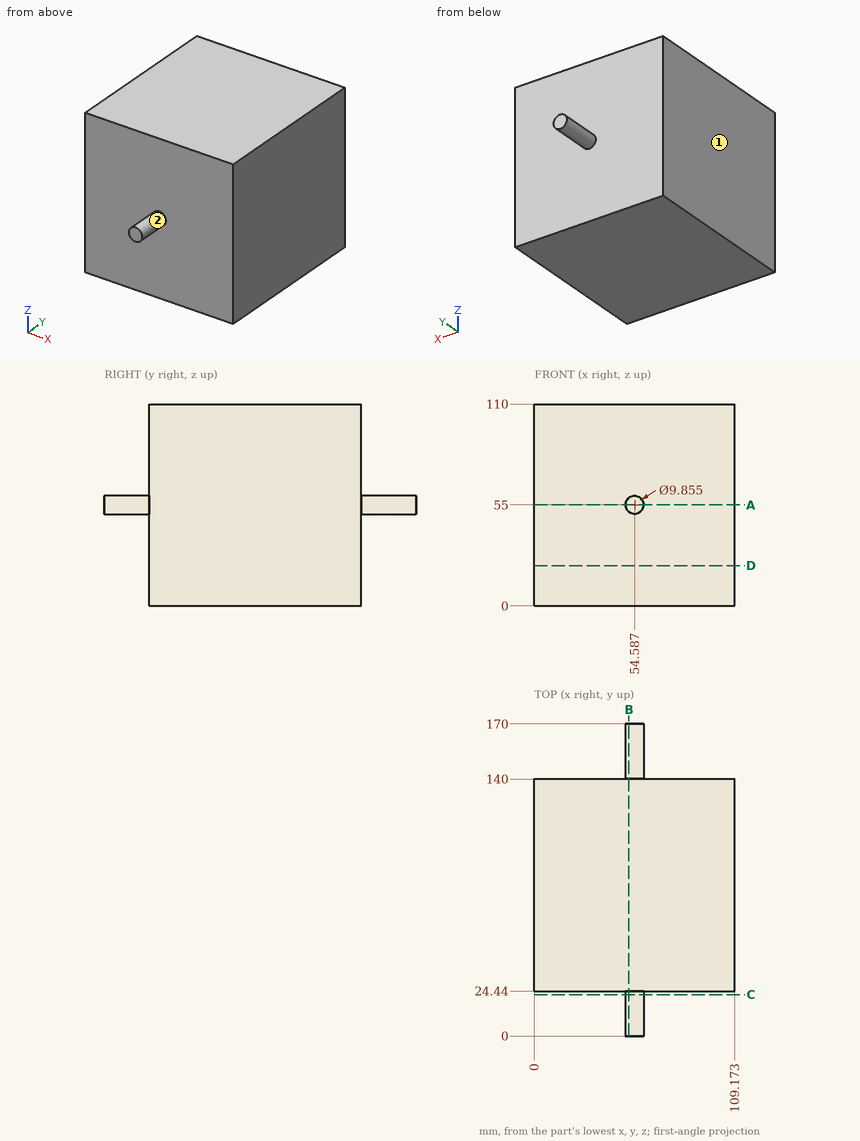
Geometry check sheet. Reference: drawing and pictorial views, mm from the part's lowest x, y, z. A direction names the side the tool comes from. Give positions to 0.01 mm unless a question says otherwise; leave off trailing zeros. Order: outer loops, then holes, each group sorted by start corner. A loop starts at its lowest first (then second) coordinate and runs counter-clockwise, first axis right, second up. Notation, with made-up numbers: (57, -8) -> (96, -8) arc R18 cw to (96, 0) -> close; hole circle Ø6 at (-35.5, 48.5). An arc over 180 degrees is marked (long way). Write each question's results on one line, items separated by ' | '. Start each with the question number.
(1) Sectioned sample at D-D (z = 22). Enter the section's corners in (x, y).
(2) Sectioned sample at A-A (z = 55). Enter the section's corners in (x, y).
(3) Gauge pin test, flat ends, axial feed: P1, Ø6, axis at x = 33, z = 26, coming from the -Y side; P2, Ø1, axis at y = 146, z = 60, coming from the +X side (1 decimal). Record the tip position at first contact, or that the pin passes through.
(4) Access from +Z, -Z, +X, -X, +Y, -Y to the whole of each face (thin tool, end or side, straight path). Record for the marked faces 1 and 2.
(5) Sectioned sample at B-B (x = 51.5). Enter the section's corners in (y, z).
(6) Scan line: line 1 (Y direction, x = 102, z = 51.5). Record every from-to range of solid material in increasing order.
(7) Sectioned sample at C-C (y = 22.5). Enter the section's corners in (x, z) (1 decimal).
Answer below:
1) outline: (0, 24.44) -> (109.17, 24.44) -> (109.17, 140) -> (0, 140) -> close
2) outline: (0, 24.44) -> (49.66, 24.44) -> (49.66, 0) -> (59.51, 0) -> (59.51, 24.44) -> (109.17, 24.44) -> (109.17, 140) -> (59.51, 140) -> (59.51, 170) -> (49.66, 170) -> (49.66, 140) -> (0, 140) -> close
3) P1: y = 24.44 | P2: x = 56.6
4) face 1: +Z, -Z, -X, +Y, -Y | face 2: -Y
5) outline: (0, 51.16) -> (24.44, 51.16) -> (24.44, 0) -> (140, 0) -> (140, 51.16) -> (170, 51.16) -> (170, 58.84) -> (140, 58.84) -> (140, 110) -> (24.44, 110) -> (24.44, 58.84) -> (0, 58.84) -> close
6) line 1: 24.44 to 140
7) outline: circle Ø9.9 at (54.6, 55)
